Answer from the drawing. Dimensions are ordinates in mm from the lowest x, y and z of the part. A direction names the side the tool comes from. Coordinates: 2 decimals unless noted, no trailing zeros. Write each loop counter-clockwise with the first axis right and the second up, starting at its lowest first coordinate (ties: lowest second). Pieces come first, ordered by that corner, then holes. Notation, with made-up numbers: (4, 15.5) -> (55, 15.5) arc R19 cw to (55, 42.5) -> close; hole circle Ø5 at (9.25, 14.5). An arc over 180 degrees is marked (long way). Return JSON: item names as keys, results as strings.
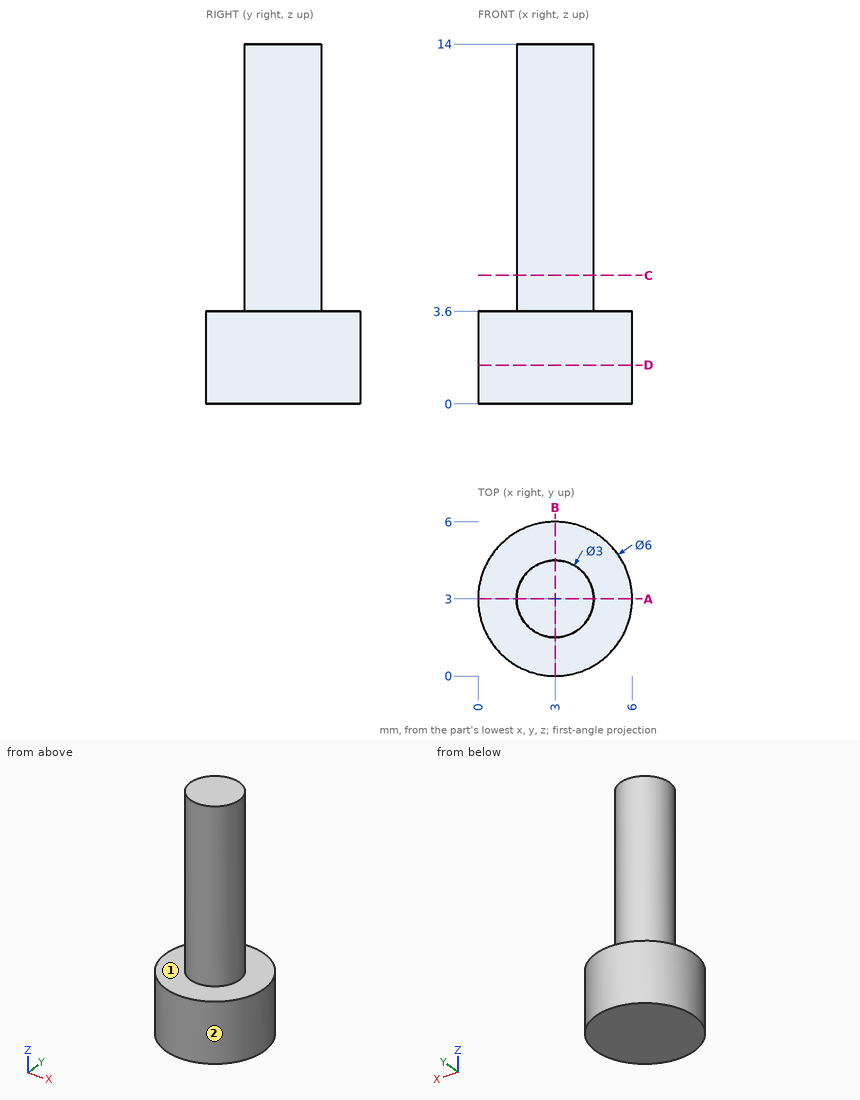
1. The part is cut by section A-A (y = 3). Determine the outline of the cut face in (x, z).
Taken from the geometry:
{"outline": "(0, 0) -> (6, 0) -> (6, 3.6) -> (4.5, 3.6) -> (4.5, 14) -> (1.5, 14) -> (1.5, 3.6) -> (0, 3.6) -> close"}
2. A tool of negligible diameter and unlimited length cuts with its end or side. For the marked faces 1 and 2, from which of +Z, -Z, +X, -X, +Y, -Y can it reach the whole face along a straight path? Write none if from no direction.
Taken from the geometry:
{"face 1": "+Z", "face 2": "+Z, -Z"}
3. The part is cut by section C-C (z = 5). Determine the outline of the cut face in (x, y).
Taken from the geometry:
{"outline": "circle Ø3 at (3, 3)"}
4. The part is cut by section D-D (z = 1.5). Determine the outline of the cut face in (x, y).
Taken from the geometry:
{"outline": "circle Ø6 at (3, 3)"}
5. Flat-ended cylindrical pins translate along their axes: pin 1 Ø3 at (y, z) = (1, 1.5) entering from +X; pin 2 Ø3 at (x, y) = (3, 2) entering from -Z; pin 3 Ø1 at (x, z) = (4, 7.5) entering from -Y. Find the tip coordinate at first contact, or state that the pin passes through.
Taken from the geometry:
{"pin 1": "stops at x = 5.96", "pin 2": "stops at z = 0", "pin 3": "stops at y = 1.59"}
6. Consider L1, parallel to Z at x = 4.9, y = 5.2; L2, parallel to Y at x = 3.6, z = 8.25. Determine where each line is inside the solid, lowest interval first.
Taken from the geometry:
{"L1": "z = 0 to 3.6", "L2": "y = 1.63 to 4.37"}
